```python
from build123d import *

# Parameters (mm, degrees)
BOSS_EXTRUDE1_DEPTH = 1.6
SKETCH2_W           = 1
SKETCH2_H           = 1
BOSS_EXTRUDE2_DEPTH = 0.3
SKETCH3_R           = 3.25
CUT_EXTRUDE1_DEPTH  = 50.108273234


with BuildPart() as part:
    # Sketch1 → Boss-Extrude1 (new body)
    with BuildSketch(Plane(origin=(0, 0, 0), x_dir=(1, 0, 0), z_dir=(0, 1, 0))):
        with BuildLine():
            Line((-45, 10.25), (45, 10.25))
            ThreePointArc((45, 10.25), (47.121320344, 9.371320344), (48, 7.25))
            Line((48, 7.25), (48, -7.25))
            ThreePointArc((48, -7.25), (47.121320344, -9.371320344), (45, -10.25))
            Line((45, -10.25), (-45, -10.25))
            ThreePointArc((-45, -10.25), (-47.121320344, -9.371320344), (-48, -7.25))
            Line((-48, -7.25), (-48, 7.25))
            ThreePointArc((-48, 7.25), (-47.121320344, 9.371320344), (-45, 10.25))
        make_face()
    extrude(amount=BOSS_EXTRUDE1_DEPTH)

    # Sketch2 → Boss-Extrude2 (add)
    with BuildSketch(Plane(origin=(0, 1.6, 0), x_dir=(1, 0, 0), z_dir=(0, 1, 0))):
        with Locations((35, 0)):
            Rectangle(SKETCH2_W, SKETCH2_H)
    extrude(amount=BOSS_EXTRUDE2_DEPTH)

    # Sketch3 → Cut-Extrude1 (cut, through all)
    with BuildSketch(Plane(origin=(0, 1.6, 0), x_dir=(1, 0, 0), z_dir=(0, 1, 0))):
        with Locations(Location((-20, 0, 0), (0, 0, 270))):
            Circle(SKETCH3_R)
    extrude(amount=-CUT_EXTRUDE1_DEPTH, mode=Mode.SUBTRACT)


solid = part.part
```
The model under review builds one solid part; all positions refer to its coordinate system, in mm. Round coordinates to 2 decimals unless told otherwise and drop trailing zeros. Write each loop counter-clockwise with the first axis right and the second up, starting at its lowest first coordinate (ties: lowest second). Pieces come first, ordered by that corner, then holes. Notation, with made-up numbers: (-8, 43) - (0, 43) arc R17 ccw to (0, 72) - close; hole circle Ø5 at (-7, -25). An arc over 180 degrees is marked (long way). Answer as CSV lines item,"result". Start each with the question number.
(1) We need section C-C on z = -1.5. State the section outline as (x, y) points, plus the area to 3 significant figures.
(2) For pin 1 Ø5 at (x, z) = (-2, -7) entering from +Y, flat-tipped, find the tip position at first contact; note if it passes through.
(3) We need section D-D on x = 21.5. State the section outline as (y, z) points.
(4) We need section A-A on x = -20. State the section outline as (y, z) points.
(5) We need section B-B on y = 1.15. State the section outline as (x, z) points.
(6) To check wall thickness, follow line 1 (X direction, y = 1.2, z = 0); line 2 (Y direction, x = 35.5, z = -4.5); line 3 (X direction, y = 0.7, z = 2.5). State the ranges of each line that lie inside material, in increasing order.
Worked answers:
1,outline,"(-48, 0) - (-22.88, 0) - (-22.88, 1.6) - (-48, 1.6) - close; (-17.12, 0) - (48, 0) - (48, 1.6) - (-17.12, 1.6) - close"
1,area,"144 mm²"
2,pin 1,"y = 1.6"
3,outline,"(0, -10.25) - (1.6, -10.25) - (1.6, 10.25) - (0, 10.25) - close"
4,outline,"(0, -10.25) - (1.6, -10.25) - (1.6, -3.25) - (0, -3.25) - close; (0, 3.25) - (1.6, 3.25) - (1.6, 10.25) - (0, 10.25) - close"
5,outline,"(-48, -7.25) arc R3 ccw to (-45, -10.25) - (45, -10.25) arc R3 ccw to (48, -7.25) - (48, 7.25) arc R3 ccw to (45, 10.25) - (-45, 10.25) arc R3 ccw to (-48, 7.25) - close; hole circle Ø6.5 at (-20, 0)"
6,line 1,"-48 to -23.25, -16.75 to 48"
6,line 2,"0 to 1.6"
6,line 3,"-48 to -22.08, -17.92 to 48"
